Here's the drawing with two shaded views (mm, measured from the low corner). I have some questions. Coordinates: 2 decimals unless noted, no trailing zeros. Order: outer loops, then holes, each group sorted by start corner. A loop starts at its lowest first (then second) coordinate and runs counter-clockwise, first axis right, second up. Notation, with made-up numbers: (80.5, 3) -> (115.5, 3) arc R21 ccw to (115.5, 14) -> close; hole circle Ø4 at (36.5, -11). An arc over 180 degrees is marked (long way). Answer as a JSON object with one key per item and string values. Group by question number.
(1) I want a section at D-D, the plane y = 11.5. List the corners of the cut face in (x, z) for me, plus the area to 3 significant figures.
(2) I want a section at C-C, the plane y = 19.05. List the corners of the cut face in (x, z) for me.
(3) I need wall thicknesses on line 1 (Y direction, x = 95.25, z = 5); line 2 (X direction, y = 19.05, z = 2.25); line 3 (X direction, y = 26.5, z = 2.5) (1 decimal). Which ranges of each line are inside material? Lowest first, please.
(4) I want a section at A-A, the plane x = 95.25. List the corners of the cut face in (y, z) for me.
(5) For pin 1 (2 mm diameter, centred on y = 5.5, z = 2.5, fed in from -X); pin 2 (12 mm diameter, centred on x = 17, y = 20, fed in from -Z), each with a flat end and sliding along its axis, tell me the tip position at first contact or that it passes through.
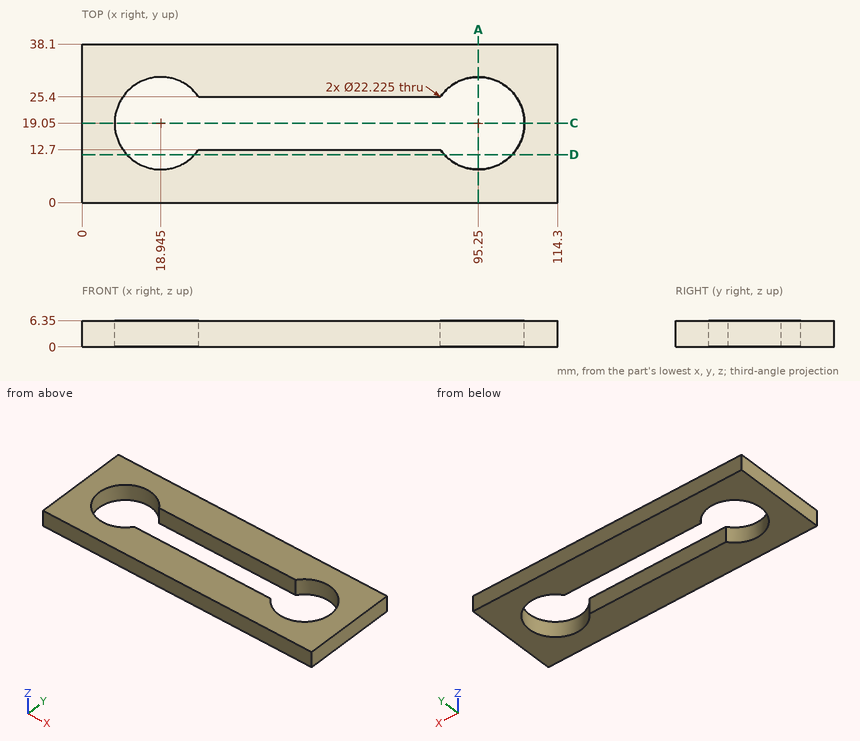
Computed values:
{
 "1": {"outline": "(0, 0) -> (10.79, 0) -> (10.79, 6.35) -> (0, 6.35) -> close; (27.1, 0) -> (87.1, 0) -> (87.1, 6.35) -> (27.1, 6.35) -> close; (103.4, 0) -> (114.3, 0) -> (114.3, 6.35) -> (103.4, 6.35) -> close", "area": "519 mm2"},
 "2": {"outline": "(0, 0) -> (7.83, 0) -> (7.83, 6.35) -> (0, 6.35) -> close; (106.36, 0) -> (114.3, 0) -> (114.3, 6.35) -> (106.36, 6.35) -> close"},
 "3": {"line 1": "y = 0 to 7.94, 30.16 to 38.1", "line 2": "x = 0 to 7.83, 106.36 to 114.3", "line 3": "x = 0 to 10.7, 27.2 to 87, 103.5 to 114.3"},
 "4": {"outline": "(0, 0) -> (7.94, 0) -> (7.94, 6.35) -> (0, 6.35) -> close; (30.16, 0) -> (38.1, 0) -> (38.1, 6.35) -> (30.16, 6.35) -> close"},
 "5": {"pin 1": "stops at x = 0", "pin 2": "passes through"}
}
